Could you check a few things on this model? Use its own coordinates, in mm. A direction names the side the tool comes from. Round coordinates to 2 decimals unless told otherwise and drop trailing zeros. Write each loop counter-clockwise with the first axis right and the second up, starting at its lowest first coordinate (ties: lowest second). Pieces come first, ordered by that corner, then holes. Notation, with made-up numbers: (73.5, 19) - (109.5, 19) arc R11 ccw to (109.5, 26) - close; hole circle Ø4 at (-0.5, 76.5). An arc over 180 degrees is marked (long way). Write each question's results on one line, items separated by ' | '. Start each with the question number.
(1) For P1, Ø1.5, axis at x = 4, z = 2, coming from the -Y side; P2, Ø1.5, axis at x = -3.5, z = 0, coming from the -Y side; P3, Ø1.5, axis at x = -5, z = 2.5, coming from the -Y side, each with a flat end and sliding along its axis, tell me the tip position at first contact or that it passes through.
(2) Imagine slicing it at C-C on z = -2.5. Write out the boundary of the cut face in (x, y), then the cut area to 3 significant figures.
(3) Thinking about a two-plate mould opening in Y: for faces 1 (the flat face through (4, 0, -7)), 2 (the cylindrical face through (-1.107, -8.428, -1.014)), 3 (the cylindrical face through (0, -4, 0)), 4 (the cylindrical face through (0, 4, 0)), which applies, +Y half, -Y half, draft (parallel to the pull), parting line (faces both ways), or undercut?
(4) On a 3-axis mill with a long thin cutter (end or side, diameter ignored), from which of +Z, -Z, +X, -X, +Y, -Y can I reach the whole of each face in a straight line? I mean faces 5 (the flat face through (-4, 0, 6)), 6 (the flat face through (-3.5, 0, 0)), 7 (the cylindrical face through (1.67, 7.47, -4.46)), 8 (the cylindrical face through (5.93, -2.87, 2.96)). Say none if no direction works.
(5) Please list where these lines run through material, in increasing order: line 1 (Y direction, x = -1.5, z = 2.5); line 2 (X direction, y = -0.5, z = 2.25); line 3 (Z direction, x = -3.5, y = 7). Write a range as [from, to].
(6) Imagine slicing it at D-D on x = -5.5. Write out the boundary of the cut face in (y, z), then the cut area to 3 significant figures.
(7) Imagine slicing it at A-A on x = 0. Write out the boundary of the cut face in (y, z).
```python
from build123d import *

# Parameters (mm, degrees)
SKETCH1_R           = 7.5
BOSS_EXTRUDE1_DEPTH = 6
SKETCH2_R           = 7.5
BOSS_EXTRUDE2_DEPTH = 7
CUT_EXTRUDE1_DEPTH  = 14.322912594
BOSS_EXTRUDE3_START = 2
SKETCH4_R           = 8.5
BOSS_EXTRUDE3_DEPTH = 2


with BuildPart() as part:
    # Sketch1 → Boss-Extrude1 (new body)
    with BuildSketch(Plane.XY):
        with Locations((-1, 0)):
            Circle(SKETCH1_R)
        with BuildLine():
            Line((3.5, -1.936491673), (3.5, 1.936491673))
            ThreePointArc((3.5, 1.936491673), (0, 4), (-3.5, 1.936491673))
            Line((-3.5, 1.936491673), (-3.5, -1.936491673))
            ThreePointArc((-3.5, -1.936491673), (0, -4), (3.5, -1.936491673))
        make_face(mode=Mode.SUBTRACT)
    extrude(amount=BOSS_EXTRUDE1_DEPTH)

    # Sketch2 → Boss-Extrude2 (add)
    with BuildSketch(Plane(origin=(0, 0, 0), x_dir=(-1, 0, 0), z_dir=(0, 0, -1))):
        with Locations(Location((-1, 0, 0), (0, 0, 277.662255661))):
            Circle(SKETCH2_R)
    extrude(amount=BOSS_EXTRUDE2_DEPTH)

    # Sketch3 → Cut-Extrude1 (cut, through all)
    with BuildSketch(Plane.XY):
        with BuildLine():
            Line((3.5, -1.936491673), (3.5, 1.936491673))
            ThreePointArc((3.5, 1.936491673), (0, 4), (-3.5, 1.936491673))
            Line((-3.5, 1.936491673), (-3.5, -1.936491673))
            ThreePointArc((-3.5, -1.936491673), (0, -4), (3.5, -1.936491673))
        make_face()
    extrude(amount=-CUT_EXTRUDE1_DEPTH, mode=Mode.SUBTRACT)

    # Sketch4 → Boss-Extrude3 (add)
    with BuildSketch(Plane(origin=(0, 0, 0), x_dir=(-1, 0, 0), z_dir=(0, 0, -1)).offset(BOSS_EXTRUDE3_START)):
        with Locations(Location((0, 0, 0), (0, 0, 180.00076113))):
            Circle(SKETCH4_R)
        with BuildLine():
            Line((3.5, 1.936491673), (3.5, -1.936491673))
            ThreePointArc((3.5, -1.936491673), (0, -4), (-3.5, -1.936491673))
            Line((-3.5, -1.936491673), (-3.5, 1.936491673))
            ThreePointArc((-3.5, 1.936491673), (0, 4), (3.5, 1.936491673))
        make_face(mode=Mode.SUBTRACT)
    extrude(amount=-BOSS_EXTRUDE3_DEPTH)


solid = part.part
```
Response:
1) P1: y = -6.18 | P2: y = -8.04 | P3: y = -6.76
2) outline: circle Ø15 at (1, 0); hole (-3.5, -1.94) arc R4 ccw to (3.5, -1.94) - (3.5, 1.94) arc R4 ccw to (-3.5, 1.94) - close | area: 129 mm²
3) face 1: draft | face 2: parting line | face 3: undercut | face 4: undercut
4) face 5: +Z, +X, -X, +Y, -Y | face 6: +Z, -Z | face 7: -Z | face 8: +Z
5) line 1: [-7.48, -3.71], [3.71, 7.48] | line 2: [-8.48, -3.5], [3.5, 6.48] | line 3: [-2, 6]
6) outline: (-6.48, -2) - (-3.74, -2) - (-3.74, -7) - (3.74, -7) - (3.74, -2) - (6.48, -2) - (6.48, 0) - (6, 0) - (6, 6) - (-6, 6) - (-6, 0) - (-6.48, 0) - close | area: 135 mm²
7) outline: (-8.5, -2) - (-7.43, -2) - (-7.43, -7) - (-4, -7) - (-4, 6) - (-7.43, 6) - (-7.43, 0) - (-8.5, 0) - close; (4, -7) - (7.43, -7) - (7.43, -2) - (8.5, -2) - (8.5, 0) - (7.43, 0) - (7.43, 6) - (4, 6) - close
